Check sheet for the drawn part. Datum: minimum x, y, z corner. Units: mm. A direction names the side the tool comes from. Give positions to 0.01 mm unless a question says otherwise; leave off trailing zeros. Loops run counter-clockwise (first coordinate to the right, second up) from the corner with the lowest first, then second, coordinate; pieces in that order, holes last.
1. Tool access check on the marked faces 1 and 2. Record the directions out of +Z, -Z, +X, -X, +Y, -Y that give a thin tool (end or side, any length) a straight path to the whole face; none if there is none.
2. Cross-section at A-A, the plane z = 7.5. Record the cut outline in (x, y).
3. Material ranges on L1, parallel to X at y = 1.7, z = 7.5; L2, parallel to Z at x = 9, y = 6.25, recorded low to high.
4. Release check for a two-part mould opening along X. For the marked faces 3, 4, 5 and 6 record: +X half, -X half, draft (parallel to the pull), parting line (faces both ways), or undercut.
5. Cross-section at C-C, the plane y = 4. Record the cut outline in (x, z).
6. Go/stop test with flat-tipped pins: pin 1 Ø2 at (x, y) = (10.5, 5) entering from -Z; pin 2 Ø1.5 at (x, y) = (9.5, 4) entering from +Z; pin 3 Ø4 at (x, y) = (12.5, 1) entering from +Z. Record where each tip stops, or that it passes through.
7. Cross-section at B-B, the plane x = 7.5. Record the cut outline in (y, z).
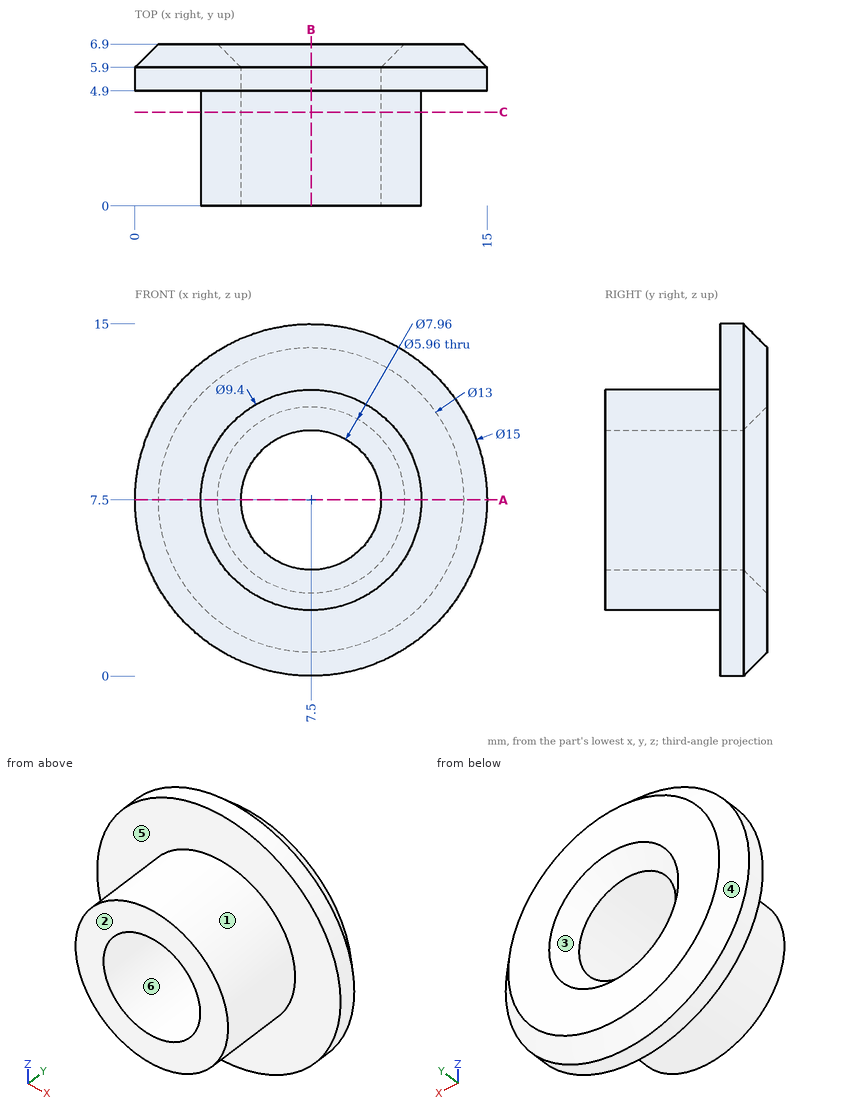
Result:
1. face 1: -Y
1. face 2: +Z, -Z, +X, -X, -Y
2. outline: (0, 4.9) - (2.8, 4.9) - (2.8, 0) - (4.52, 0) - (4.52, 5.9) - (3.52, 6.9) - (1, 6.9) - (0, 5.9) - close; (10.48, 0) - (12.2, 0) - (12.2, 4.9) - (15, 4.9) - (15, 5.9) - (14, 6.9) - (11.48, 6.9) - (10.48, 5.9) - close
3. L1: x = 2.8 to 4.52, 10.48 to 12.2
3. L2: z = 0.51 to 4.53, 10.47 to 14.49
4. face 3: undercut
4. face 4: parting line
4. face 5: draft
4. face 6: undercut
5. outline: circle Ø9.4 at (7.5, 7.5); hole circle Ø5.96 at (7.5, 7.5)
6. pin 1: stops at z = 0.27
6. pin 2: stops at z = 12.03
6. pin 3: stops at z = 11.12
7. outline: (0, 2.8) - (4.9, 2.8) - (4.9, 0) - (5.9, 0) - (6.9, 1) - (6.9, 3.52) - (5.9, 4.52) - (0, 4.52) - close; (0, 10.48) - (5.9, 10.48) - (6.9, 11.48) - (6.9, 14) - (5.9, 15) - (4.9, 15) - (4.9, 12.2) - (0, 12.2) - close
